Could you check a few things on this model? Use its own coordinates, in mm. A direction names the side the tool comes from. Coordinates: 2 decimals unless noted, no trailing zeros. Loops run counter-clockwise (first coordinate to the right, second up) from the corner with the lowest first, then second, coordinate; pieces in that order, holes last. Notation, with made-up numbers: (40, 64) - (78, 64) arc R27 ccw to (78, 98) - close; hole circle Ø11 at (-15.5, 80.25). An arc over 180 degrees is marked (long way). Put each result on its own line as item: value. Start each with the question number.
```python
from build123d import *

# Parameters (mm, degrees)
SKETCH_1_R           = 41
SKETCH_1_R_2         = 39
EXTRUDE_1_DEPTH      = 20
EXTRUDE_START        = -14
EXTRUDE_2_DEPTH      = 14
EXTRUDE_START_2      = -3
SKETCH_3_R           = 4
SKETCH_3_R_2         = 1.6
EXTRUDE_3_DEPTH      = 3
CUT_EXTRUDE_3_DEPTH  = 3
EXTRUDE_5_DEPTH      = 10
EXTRUDE_5_DEPTH_BACK = 15
SKETCH_1_2_R         = 41
SKETCH_1_2_R_2       = 39
EXTRUDE_START_3      = 10
EXTRUDE_7_DEPTH      = 10
EXTRUDE_8_DEPTH      = 10
EXTRUDE_8_DEPTH_BACK = 5
CUT_EXTRUDE_4_DEPTH  = 10
EXTRUDE_9_DEPTH      = 10
EXTRUDE_9_DEPTH_BACK = 1.5
CUT_EXTRUDE_6_DEPTH  = 10
SKETCH_16_R          = 1.6
CUT_EXTRUDE_7_DEPTH  = 3
SKETCH_18_R          = 1.6
CUT_EXTRUDE_8_DEPTH  = 10
SKETCH_18_4_R        = 1.6
CUT_EXTRUDE_9_DEPTH  = 10


with BuildPart() as part:
    # Sketch 1 → Extrude 1 (new body)
    with BuildSketch(Plane(origin=(0, 0, 0), x_dir=(1, 0, 0), z_dir=(0, 1, 0))):
        with Locations(Location((0, 0, 0), (0, 0, 270))):
            Circle(SKETCH_1_R)
        with Locations(Location((0, 0, 0), (0, 0, 270))):
            Circle(SKETCH_1_R_2, mode=Mode.SUBTRACT)
    extrude(amount=EXTRUDE_1_DEPTH)

    # Sketch 2 → Extrude 2 (add)
    with BuildSketch(Plane(origin=(0, 20, 0), x_dir=(1, 0, 0), z_dir=(0, 1, 0)).offset(EXTRUDE_START)):
        with BuildLine():
            Line((-20, -41), (3.5e-08, -41))
            ThreePointArc((3.5e-08, -41), (-10.333598732, -39.676400256), (-20, -35.791060336))
            Line((-20, -35.791060336), (-20, -41))
        make_face()
        with BuildLine():
            Line((3.5e-08, -41), (20, -41))
            Line((20, -41), (20, -35.791060336))
            ThreePointArc((20, -35.791060336), (10.333598766, -39.676400247), (3.5e-08, -41))
        make_face()
    extrude(amount=EXTRUDE_2_DEPTH)

    # Sketch 3 → Extrude 3 (add)
    with BuildSketch(Plane(origin=(0, 20, 0), x_dir=(1, 0, 0), z_dir=(0, 1, 0)).offset(EXTRUDE_START_2)):
        with BuildLine():
            Line((-2, 38.948684188), (-2, 11.324751653))
            ThreePointArc((-2, 11.324751653), (-9.959292144, 5.75), (-10.807522623, -3.930325019))
            Line((-10.807522623, -3.930325019), (-34.730549951, -17.742291287))
            ThreePointArc((-34.730549951, -17.742291287), (-33.774990748, -19.5), (-32.730549951, -21.206392902))
            Line((-32.730549951, -21.206392902), (-8.807522623, -7.394426634))
            ThreePointArc((-8.807522623, -7.394426634), (0, -11.5), (8.807522623, -7.394426634))
            Line((8.807522623, -7.394426634), (32.730549951, -21.206392902))
            ThreePointArc((32.730549951, -21.206392902), (33.774990748, -19.5), (34.730549951, -17.742291287))
            Line((34.730549951, -17.742291287), (10.807522623, -3.930325019))
            ThreePointArc((10.807522623, -3.930325019), (9.959292144, 5.75), (2, 11.324751653))
            Line((2, 11.324751653), (2, 38.948684188))
            ThreePointArc((2, 38.948684188), (0, 39), (-2, 38.948684188))
        make_face()
        with Locations(Location((0, 0, 0), (0, 0, 270))):
            Circle(SKETCH_3_R, mode=Mode.SUBTRACT)
        with Locations(Location((-8, 0, 0), (0, 0, 270))):
            Circle(SKETCH_3_R_2, mode=Mode.SUBTRACT)
        with Locations(Location((8, 0, 0), (0, 0, 270))):
            Circle(SKETCH_3_R_2, mode=Mode.SUBTRACT)
    extrude(amount=EXTRUDE_3_DEPTH)

    # Sketch 7 → Cut-Extrude 3 (cut)
    with BuildSketch(Plane.XZ.offset(-6)):
        with BuildLine():
            Line((0, 41), (-20, 41))
            Line((-20, 41), (-20, 35.791060336))
            ThreePointArc((-20, 35.791060336), (-10.333598749, 39.676400251), (0, 41))
        make_face()
        with BuildLine():
            Line((20, 41), (0, 41))
            ThreePointArc((0, 41), (10.333598749, 39.676400251), (20, 35.791060336))
            Line((20, 35.791060336), (20, 41))
        make_face()
    extrude(amount=-CUT_EXTRUDE_3_DEPTH, mode=Mode.SUBTRACT)

    # Sketch 1_2 → Extrude 5 (add, two sides: drawn at the far end of the back side and taken through both)
    with BuildSketch(Plane(origin=(0, 0, 0), x_dir=(1, 0, 0), z_dir=(0, 1, 0)).offset(-EXTRUDE_5_DEPTH_BACK)):
        with Locations(Location((0, 0, 0), (0, 0, 270))):
            Circle(SKETCH_1_2_R)
        with Locations(Location((0, 0, 0), (0, 0, 92.939534486))):
            Circle(SKETCH_1_2_R_2, mode=Mode.SUBTRACT)
    extrude(amount=EXTRUDE_5_DEPTH + EXTRUDE_5_DEPTH_BACK)

    # Sketch 7_4 → Extrude 7 (add)
    with BuildSketch(Plane.XZ.offset(-6).offset(EXTRUDE_START_3)):
        with BuildLine():
            Line((0, 41), (-20, 41))
            Line((-20, 41), (-20, 35.791060336))
            ThreePointArc((-20, 35.791060336), (-10.333598749, 39.676400251), (0, 41))
        make_face()
        with BuildLine():
            Line((20, 41), (0, 41))
            ThreePointArc((0, 41), (10.333598749, 39.676400251), (20, 35.791060336))
            Line((20, 35.791060336), (20, 41))
        make_face()
    extrude(amount=-EXTRUDE_7_DEPTH)

    # Sketch 7_5 → Extrude 8 (add, two sides: drawn at the far end of the back side and taken through both)
    with BuildSketch(Plane.XZ.offset(-6).offset(-EXTRUDE_8_DEPTH_BACK)):
        with BuildLine():
            Line((0, 41), (-20, 41))
            Line((-20, 41), (-20, 35.791060336))
            ThreePointArc((-20, 35.791060336), (-10.333598749, 39.676400251), (0, 41))
        make_face()
        with BuildLine():
            Line((20, 41), (0, 41))
            ThreePointArc((0, 41), (10.333598749, 39.676400251), (20, 35.791060336))
            Line((20, 35.791060336), (20, 41))
        make_face()
    extrude(amount=EXTRUDE_8_DEPTH + EXTRUDE_8_DEPTH_BACK)

    # Sketch 4 → Cut-Extrude 4 (cut)
    with BuildSketch(Plane.XY.offset(41)):
        Polygon((-10, 4.766838493), (-7.2, 6.383419246), (-7.2, 9.616580754), (-10, 11.233161507), (-12.8, 9.616580754), (-12.8, 6.383419246), align=None)
        Polygon((12.8, 6.383419246), (10, 4.766838493), (7.2, 6.383419246), (7.2, 9.616580754), (10, 11.233161507), (12.8, 9.616580754), align=None)
    extrude(amount=-CUT_EXTRUDE_4_DEPTH, mode=Mode.SUBTRACT)

    # Sketch 4_3 → Extrude 9 (add, two sides: drawn at the far end of the back side and taken through both)
    with BuildSketch(Plane.XY.offset(41).offset(-EXTRUDE_9_DEPTH_BACK)):
        Polygon((-10, 4.766838493), (-7.2, 6.383419246), (-7.2, 9.616580754), (-10, 11.233161507), (-12.8, 9.616580754), (-12.8, 6.383419246), align=None)
        Polygon((12.8, 6.383419246), (10, 4.766838493), (7.2, 6.383419246), (7.2, 9.616580754), (10, 11.233161507), (12.8, 9.616580754), align=None)
    extrude(amount=EXTRUDE_9_DEPTH + EXTRUDE_9_DEPTH_BACK)

    # Sketch 13 → Cut-Extrude 6 (cut)
    with BuildSketch(Plane.XY.offset(51)):
        Polygon((10, 11.233161507), (7.2, 9.616580754), (7.2, 6.383419246), (10, 4.766838493), (12.8, 6.383419246), (12.8, 9.616580754), align=None)
        Polygon((-10, 11.233161507), (-12.8, 9.616580754), (-12.8, 6.383419246), (-10, 4.766838493), (-7.2, 6.383419246), (-7.2, 9.616580754), align=None)
    extrude(amount=-CUT_EXTRUDE_6_DEPTH, mode=Mode.SUBTRACT)

    # Sketch 16 → Cut-Extrude 7 (cut)
    with BuildSketch(Plane.XY.offset(41)):
        with Locations((-10, 8)):
            Circle(SKETCH_16_R)
        with Locations(Location((10, 8, 0), (0, 0, 180))):
            Circle(SKETCH_16_R)
    extrude(amount=-CUT_EXTRUDE_7_DEPTH, mode=Mode.SUBTRACT)

    # Sketch 18 → Cut-Extrude 8 (cut)
    with BuildSketch(Plane(origin=(0, 20, 0), x_dir=(1, 0, 0), z_dir=(0, 1, 0))):
        with Locations(Location((0, 8, 0), (0, 0, 270))):
            Circle(SKETCH_18_R)
    extrude(amount=-CUT_EXTRUDE_8_DEPTH, mode=Mode.SUBTRACT)

    # Sketch 18_4 → Cut-Extrude 9 (cut)
    with BuildSketch(Plane(origin=(0, 20, 0), x_dir=(1, 0, 0), z_dir=(0, 1, 0))):
        with Locations(Location((0, 8, 0), (0, 0, 270))):
            Circle(SKETCH_18_4_R)
        with Locations(Location((0, -8, 0), (0, 0, 270))):
            Circle(SKETCH_18_4_R)
    extrude(amount=-CUT_EXTRUDE_9_DEPTH, mode=Mode.SUBTRACT)


solid = part.part
```
(1) I want a section at C-C on x = -15. List the corners of the cut face in (y, z) for me.
(2) If we mould it in two halves opening along X, with no side actions, what happens to faces 1 (the flat face through (-20, 8, 38)), 2 (the cylindrical face through (-0.1, 18.5, 11.5)), 3 (the flat face through (-15, -4, 40)), 4 (the cylindrical face through (0.07, 18.52, 6.4))? For each: pulls with the +X half, pulls with the -X half, needs draft (parallel to the pull), parting line crosses it, or undercut.
(3) I want a section at B-B on z = -29. List the corners of the cut face in (x, y) for me.
(4) I want a section at A-A on y = 8. List the corners of the cut face in (x, z) for me.
(5) I need wall thicknesses on L1, parallel to X at y = 17.95, z = 0; L2, parallel to X at y = 1, z = -0.5; L3, parallel to Z at x = 7, y = -5. Which ranges of each line are inside material? Lowest first, please. Write a range as [from, to].
(6) Which directions (+Z, -Z, +X, -X, +Y, -Y) give clear straight access to the entire face, cutting with the end or side of a thin tool? Please do faces 5 (the flat face through (0, 8, 41)), 6 (the flat face through (-11.42, 5.586, 38.484)), 7 (the flat face through (22.936, 18.479, 10.933)).
(7) For pin 1 Ø1.9 at (x, z) = (0, -8) entering from -Y; pin 2 Ø1.3 at (y, z) = (8.5, 39) entering from -X; pin 3 Ø4 at (x, y) = (14.5, 6) entering from -Z; pin 4 Ø8 at (x, y) = (-31.5, 8.5) entering from -Z, each with a flat end and sliding along its axis, tell me the tip position at first contact or that it passes through.
(8) I want a section at D-D on z = 23. List the corners of the cut face in (x, y) for me, and give its area (3 significant figures).
Answer sheet:
1. outline: (-15, -38.16) - (20, -38.16) - (20, -36) - (-15, -36) - close; (-15, 36) - (20, 36) - (20, 41) - (-4, 41) - (-4, 38.16) - (-15, 38.16) - close; (17, 6.35) - (20, 6.35) - (20, 10.97) - (17, 10.97) - close
2. face 1: pulls with the -X half
2. face 2: undercut
2. face 3: needs draft
2. face 4: undercut
3. outline: (-28.98, -15) - (-26.08, -15) - (-26.08, 20) - (-28.98, 20) - close; (-2, 17) - (2, 17) - (2, 20) - (-2, 20) - close; (26.08, -15) - (28.98, -15) - (28.98, 20) - (26.08, 20) - close
4. outline: (-20, 35.79) arc R41 ccw (long way) to (20, 35.79) - (20, 41) - (11.6, 41) - (11.6, 39.5) - (12.8, 39.5) - (12.8, 36.84) arc R39 cw (long way) to (-12.8, 36.84) - (-12.8, 39.5) - (-11.6, 39.5) - (-11.6, 41) - (-20, 41) - close; (-8.4, 39.5) - (-7.2, 39.5) - (-7.2, 38.33) arc R39 cw to (7.2, 38.33) - (7.2, 39.5) - (8.4, 39.5) - (8.4, 41) - (-8.4, 41) - close
5. L1: x = [-41, -39], [-11.5, -9.6], [-6.4, -4], [4, 6.4], [9.6, 11.5], [39, 41]
5. L2: x = [-41, -39], [39, 41]
5. L3: z = [-40.4, -38.37], [38.37, 40.4]
6. face 5: +Z, +X, -X, +Y, -Y
6. face 6: none
6. face 7: +Y, -Y
7. pin 1: passes through
7. pin 2: stops at x = -20
7. pin 3: stops at z = -39.05
7. pin 4: stops at z = -30.41
8. outline: (-33.94, -15) - (-31.5, -15) - (-31.5, 20) - (-33.94, 20) - close; (31.5, -15) - (33.94, -15) - (33.94, 20) - (31.5, 20) - close
8. area: 171 mm^2
